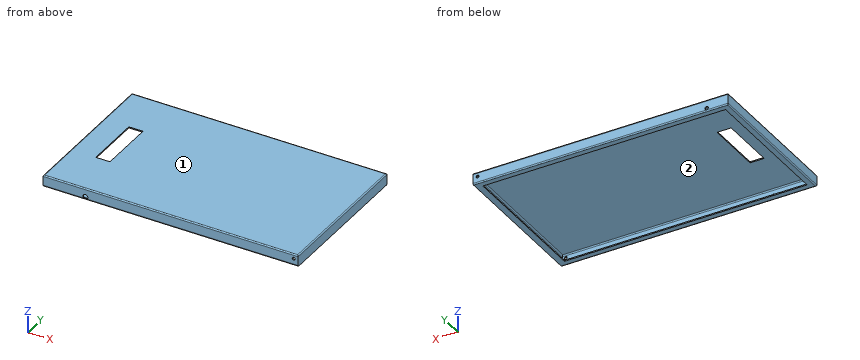
from build123d import *

# Parameters (mm, degrees)
SKETCH1_W           = 451
SKETCH1_H           = 269
BOSS_EXTRUDE1_DEPTH = 20
SHELL1_T            = -11
SKETCH2_W           = 429
SKETCH2_H           = 247
CUT_EXTRUDE1_DEPTH  = 9
SKETCH4_W           = 16
SKETCH4_H           = 247
CUT_EXTRUDE3_DEPTH  = 9
SKETCH8_W           = 438
SKETCH8_H           = 16
CUT_EXTRUDE4_DEPTH  = 9
SKETCH9_W           = 16
SKETCH9_H           = 256
CUT_EXTRUDE5_DEPTH  = 9
SKETCH10_W          = 447
SKETCH10_H          = 16
CUT_EXTRUDE6_DEPTH  = 9
SKETCH11_W          = 25
SKETCH11_H          = 100
CUT_EXTRUDE7_DEPTH  = 2
FILLET1_R           = 2
FILLET2_R           = 2
SKETCH12_R          = 3
CUT_EXTRUDE8_DEPTH  = 2
SKETCH13_R          = 4.399472723
CUT_EXTRUDE9_DEPTH  = 2
SKETCH14_R          = 2.5
CUT_EXTRUDE10_DEPTH = 270


with BuildPart() as part:
    # Sketch1 → Boss-Extrude1 (new body)
    with BuildSketch(Plane.XY):
        Rectangle(SKETCH1_W, SKETCH1_H)
    extrude(amount=BOSS_EXTRUDE1_DEPTH)

    # Shell1
    shell1_openings = [part.faces().sort_by_distance(p)[0] for p in [
        (0, 0, 0),
    ]]
    offset(amount=SHELL1_T, openings=shell1_openings, kind=Kind.INTERSECTION)

    # Sketch2 → Cut-Extrude1 (cut)
    with BuildSketch(Plane(origin=(0, 0, 9), x_dir=(-1, 0, 0), z_dir=(0, 0, -1))):
        Rectangle(SKETCH2_W, SKETCH2_H)
    extrude(amount=-CUT_EXTRUDE1_DEPTH, mode=Mode.SUBTRACT)

    # Sketch4 → Cut-Extrude3 (cut)
    with BuildSketch(Plane.ZY.offset(-214.5)):
        with Locations((10, 0)):
            Rectangle(SKETCH4_W, SKETCH4_H)
    extrude(amount=-CUT_EXTRUDE3_DEPTH, mode=Mode.SUBTRACT)

    # Sketch8 → Cut-Extrude4 (cut)
    with BuildSketch(Plane.XZ.offset(-123.5)):
        with Locations((4.5, 10)):
            Rectangle(SKETCH8_W, SKETCH8_H)
    extrude(amount=-CUT_EXTRUDE4_DEPTH, mode=Mode.SUBTRACT)

    # Sketch9 → Cut-Extrude5 (cut)
    with BuildSketch(Plane(origin=(-214.5, 0, 0), x_dir=(0, 0, -1), z_dir=(1, 0, 0))):
        with Locations((-10, 4.5)):
            Rectangle(SKETCH9_W, SKETCH9_H)
    extrude(amount=-CUT_EXTRUDE5_DEPTH, mode=Mode.SUBTRACT)

    # Sketch10 → Cut-Extrude6 (cut)
    with BuildSketch(Plane(origin=(0, -123.5, 0), x_dir=(1, 0, 0), z_dir=(0, 1, 0))):
        with Locations((0, -10)):
            Rectangle(SKETCH10_W, SKETCH10_H)
    extrude(amount=-CUT_EXTRUDE6_DEPTH, mode=Mode.SUBTRACT)

    # Sketch11 → Cut-Extrude7 (cut)
    with BuildSketch(Plane.XY.offset(20)):
        with Locations((-169, 0)):
            Rectangle(SKETCH11_W, SKETCH11_H)
    extrude(amount=-CUT_EXTRUDE7_DEPTH, mode=Mode.SUBTRACT)

    # Fillet1
    fillet1_edges = [part.edges().sort_by_distance(p)[0] for p in [
        (-225.5, 0, 20),
        (0, -134.5, 20),
        (223.5, 0, 2),
        (225.5, 0, 20),
        (0, -134.5, 0),
        (-225.5, 0, 0),
        (0, 134.5, 0),
        (0, 134.5, 20),
    ]]
    fillet(fillet1_edges, radius=FILLET1_R)

    # Fillet2
    fillet2_edges = [part.edges().sort_by_distance(p)[0] for p in [
        (223.5, 0, 18),
        (0, 132.5, 18),
        (-223.5, 0, 18),
        (0, -132.5, 18),
    ]]
    fillet(fillet2_edges, radius=FILLET2_R)

    # Sketch12 → Cut-Extrude8 (cut)
    with BuildSketch(Plane(origin=(0, 134.5, 0), x_dir=(1, 0, 0), z_dir=(0, 1, 0))):
        with Locations((-187.5, -5)):
            Circle(SKETCH12_R)
    extrude(amount=-CUT_EXTRUDE8_DEPTH, mode=Mode.SUBTRACT)

    # Sketch13 → Cut-Extrude9 (cut)
    with BuildSketch(Plane.XZ.offset(134.5)):
        with Locations((-150.5, 5)):
            Circle(SKETCH13_R)
    extrude(amount=-CUT_EXTRUDE9_DEPTH, mode=Mode.SUBTRACT)

    # Sketch14 → Cut-Extrude10 (cut, through all)
    with BuildSketch(Plane.XZ.offset(134.5)):
        with Locations((217.5, 12)):
            Circle(SKETCH14_R)
    extrude(amount=-CUT_EXTRUDE10_DEPTH, mode=Mode.SUBTRACT)


solid = part.part
Geometry: final body of the model. Coordinates: model frame, mm. Face numbers are marked on the shaded views. Give positions to 0.01 mm unless a question says otherwise; leave off trailing zeros. Write each loop counter-clockwise with the first axis right and the second up, starting at its lowest first coordinate (ties: lowest second). Pieces come first, ordered by that corner, then holes. Notation, with made-up numbers: (60.25, -31) -> (88.25, -31) arc R21 cw to (88.25, -25) -> close; hole circle Ø8 at (58.25, -11.75). An arc over 180 degrees is marked (long way). Answer as a JSON object with one key per item and string values.
1. Cut plane A-A on y = 29. Output: boundary loops of the cut face in (x, z).
Ans:
{"outline": "(-225.5, 2) arc R2 ccw to (-223.5, 0) -> (-214.5, 0) -> (-214.5, 2) -> (-223.5, 2) -> (-223.5, 16) arc R2 cw to (-221.5, 18) -> (-181.5, 18) -> (-181.5, 20) -> (-223.5, 20) arc R2 ccw to (-225.5, 18) -> close; (-156.5, 18) -> (221.5, 18) arc R2 cw to (223.5, 16) -> (223.5, 4) arc R2 cw to (221.5, 2) -> (214.5, 2) -> (214.5, 0) -> (225.5, 0) -> (225.5, 18) arc R2 ccw to (223.5, 20) -> (-156.5, 20) -> close"}
2. Ray query, probe 1 along Y at (x, z) = (136, 4); probe 2 along X at (y, z) = (59, 4.25); probe 3 along Z at (x, y) = (-187.5, 133.1). Return the intervals inside material, ascending. Write a range as from..to.
Ans:
{"probe 1": "y = -134.5..-132.5, 132.5..134.5", "probe 2": "x = -225.5..-223.5, 223.5..225.5", "probe 3": "z = 0.09..2, 8..19.91"}
3. Mould query, pull axis X, two halves, no side actions, for the marked faces 1 and 2. Classes: pulls with the +X half, pulls with the -X half, needs draft (parallel to the pull), parting line crosses it, or undercut.
Ans:
{"face 1": "needs draft", "face 2": "undercut"}
4. Cut plane B-B on y = 63.5. Output: boundary loops of the cut face in (x, z).
Ans:
{"outline": "(-225.5, 2) arc R2 ccw to (-223.5, 0) -> (-214.5, 0) -> (-214.5, 2) -> (-223.5, 2) -> (-223.5, 16) arc R2 cw to (-221.5, 18) -> (221.5, 18) arc R2 cw to (223.5, 16) -> (223.5, 4) arc R2 cw to (221.5, 2) -> (214.5, 2) -> (214.5, 0) -> (225.5, 0) -> (225.5, 18) arc R2 ccw to (223.5, 20) -> (-223.5, 20) arc R2 ccw to (-225.5, 18) -> close"}
5. Contact query for flat-ended pins moving along their axis: pin 1 (1 mm diameter, centred on y = 12, z = 19, fed in from -X); pin 2 (4 mm diameter, centred on x = 57, y = -74.5, fed in from -Z); pin 3 (8 mm diameter, centred on x = -150.5, z = 5, fed in from -Y). Output: stop coordinate, or through.
Ans:
{"pin 1": "stops at x = -225.44", "pin 2": "stops at z = 18", "pin 3": "stops at y = -132.5"}
6. Cut plane C-C on x = -96.5. Output: boundary loops of the cut face in (y, z).
Ans:
{"outline": "(-134.5, 2) arc R2 ccw to (-132.5, 0) -> (-123.5, 0) -> (-123.5, 2) -> (-132.5, 2) -> (-132.5, 16) arc R2 cw to (-130.5, 18) -> (130.5, 18) arc R2 cw to (132.5, 16) -> (132.5, 2) -> (123.5, 2) -> (123.5, 0) -> (132.5, 0) arc R2 ccw to (134.5, 2) -> (134.5, 18) arc R2 ccw to (132.5, 20) -> (-132.5, 20) arc R2 ccw to (-134.5, 18) -> close"}
